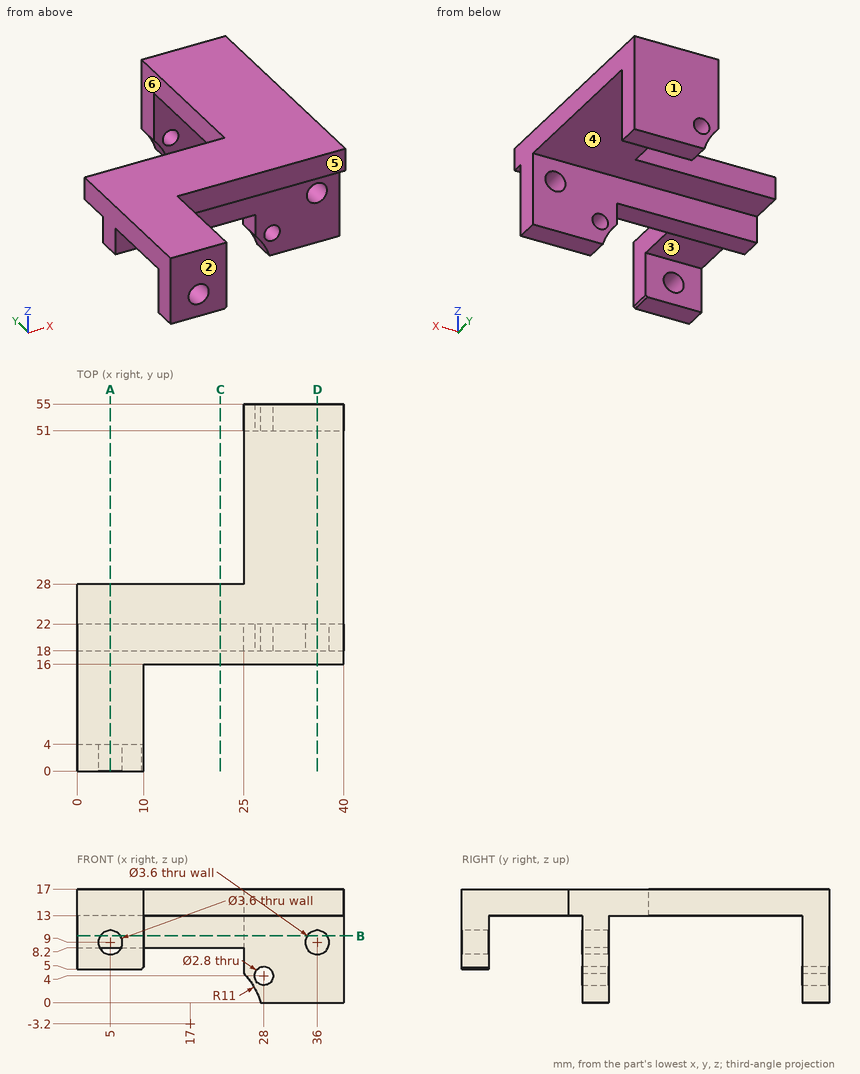
Job drawing, mm, ordinate dimensions from the low corner. One solid piece. A direction names the side the tool comes from. Round coordinates to 2 decimals unless told otherwise and drop trailing zeros. Loops run counter-clockwise (first coordinate to the right, second up) from the corner with the lowest first, then second, coordinate; pieces in that order, holes last.
Item 1: Cut at D-D, the plane x = 36. Give the cut face in (y, z), then the cut area to 3 significant figures.
Item 2: Cut at A-A, the plane x = 5. Give the cut face in (y, z), then the cut area to 3 significant figures.
Item 3: 3-axis set-ups, long thin cutter, end or side, ignore diameter. For the marked faces 4, 5 and 6: which of +Z, -Z, +X, -X, +Y, -Y reach the whole face in a straight line?
Item 4: Cut at B-B, the plane z = 10. Give the cut face in (x, y).
Item 5: Cut at C-C, the plane x = 21.5. Give the cut face in (y, z).
Item 6: Mould opens along Y. For the marked faces 1, 2 and 3 say: +Y half, -Y half, draft (parallel to the pull), parting line (faces both ways), or undercut.
Item 7: Drill centre lines: line 1 (Y direction, x = 30.5, z = 3); line 2 (Z direction, x = 5, y = 3); line 3 (Y direction, x = 11, z = 11.25). Where is each one in solid material? Low to high.
Item 8: Drop flat-ended pins along their axis: P1, Ø8, axis at x = 20.5, z = 15, coming from the -Y side; P2, Ø1.2, axis at x = 6, y = 3, coming from the -Z side; P3, Ø1.2, axis at x = 7.5, y = 20, coming from the -Z side; P4, Ø14.5, axis at x = 12.5, y = 43.5, coming from the -Z side. Give the stop position or say it passes through.
A:
1. outline: (16, 13) - (18, 13) - (18, 10.8) - (22, 10.8) - (22, 13) - (51, 13) - (51, 0) - (55, 0) - (55, 17) - (16, 17) - close; (18, 0) - (22, 0) - (22, 7.2) - (18, 7.2) - close
1. area: 246 mm2
2. outline: (0, 5) - (4, 5) - (4, 7.2) - (0, 7.2) - close; (0, 10.8) - (4, 10.8) - (4, 13) - (18, 13) - (18, 8.2) - (22, 8.2) - (22, 13) - (28, 13) - (28, 17) - (0, 17) - close
2. area: 149 mm2
3. face 4: -Z, +X, -X
3. face 5: +Z, -Z, +X, -Y
3. face 6: +Z, -Z, -X, +Y
4. outline: (0, 0) - (3.5, 0) - (3.5, 4) - (0, 4) - close; (0, 18) - (34.5, 18) - (34.5, 22) - (0, 22) - close; (6.5, 0) - (10, 0) - (10, 4) - (6.5, 4) - close; (25, 51) - (40, 51) - (40, 55) - (25, 55) - close; (37.5, 18) - (40, 18) - (40, 22) - (37.5, 22) - close
5. outline: (16, 13) - (18, 13) - (18, 8.2) - (22, 8.2) - (22, 13) - (28, 13) - (28, 17) - (16, 17) - close
6. face 1: +Y half
6. face 2: -Y half
6. face 3: undercut
7. line 1: y = 18 to 22, 51 to 55
7. line 2: z = 5 to 7.2, 10.8 to 17
7. line 3: y = 18 to 22
8. P1: stops at y = 16
8. P2: stops at z = 5
8. P3: stops at z = 8.2
8. P4: passes through
